Verification items for the finished model (mm, model axes). A direction names the side the tool comes from. Round coordinates to 2 decimals unless told otherwise and drop trailing zeros. Loops run counter-clockwise (first coordinate to the right, second up) from the corner with the lowest first, then second, coordinate; pieces in that order, holes last. Notation, with made-up numbers: (-10.5, 32.25) - (16.5, 32.25) arc R9 cw to (16.5, 40.25) - close; hole circle Ø5 at (75, 64.5). An arc over 180 degrees is marked (long way). Use CSV: the item, a comma, the result in double quotes.
```python
from build123d import *

# Parameters (mm, degrees)
F0_W     = 80
F0_H     = 19
F0_R     = 2.55
F1_DEPTH = 19
F2_R     = 5
F3_DEPTH = 4.5


with BuildPart() as f1:
    # F0 (on Top) → F1 (new body)
    with BuildSketch(Plane.XY):
        Rectangle(F0_W, F0_H)
        with Locations((-30, 0)):
            Circle(F0_R, mode=Mode.SUBTRACT)
        with Locations((-10, 0)):
            Circle(F0_R, mode=Mode.SUBTRACT)
        with Locations((10, 0)):
            Circle(F0_R, mode=Mode.SUBTRACT)
        with Locations((30, 0)):
            Circle(F0_R, mode=Mode.SUBTRACT)
    extrude(amount=F1_DEPTH)

    # F2 (on face) → F3 (cut)
    with BuildSketch(Plane.XY.offset(19)):
        with Locations((-30, 0)):
            Circle(F2_R)
        with Locations((-10, 0)):
            Circle(F2_R)
        with Locations((10, 0)):
            Circle(F2_R)
        with Locations((30, 0)):
            Circle(F2_R)
    extrude(amount=-F3_DEPTH, mode=Mode.SUBTRACT)


solid = f1.part
```
1) Mould release check, pull along X, two halves, no side actions. Record for faces 3 (the face through (-40, 0, 9)), 4 (the face through (-28, -2, 14.5)), 5 (the face through (40, 0, 9)): +X half, -X half, draft (parallel to the pull), parting line (faces both ways), or undercut.
Returned:
face 3,"-X half"
face 4,"undercut"
face 5,"+X half"
2) Cross-section at B-B, the plane z = 7. Record the cut outline in (x, y), then the cut area to 3 significant figures.
Returned:
outline,"(-40, -9.5) - (40, -9.5) - (40, 9.5) - (-40, 9.5) - close; hole circle Ø5.1 at (-30, 0); hole circle Ø5.1 at (-10, 0); hole circle Ø5.1 at (10, 0); hole circle Ø5.1 at (30, 0)"
area,"1,440 mm²"
3) Cross-section at D-D, the plane y = 0. Count the separate pieces of the cut face and the enclosed holes in it, then the cut area to 3 significant figures.
Returned:
separate pieces,"5"
enclosed holes,"0"
area,"1,040 mm²"
4) Cross-section at A-A, the plane x = 30. Record the cut outline in (y, z).
Returned:
outline,"(-9.5, 0) - (-2.55, 0) - (-2.55, 14.5) - (-5, 14.5) - (-5, 19) - (-9.5, 19) - close; (2.55, 0) - (9.5, 0) - (9.5, 19) - (5, 19) - (5, 14.5) - (2.55, 14.5) - close"
5) Access from +Z, -Z, +X, -X, +Y, -Y to the whole of each face (thin tool, end or side, straight path). Record for faces 1 (the face through (12, -2, 14.5)), 2 (the face through (27.452, 0.112, 7.148)).
Returned:
face 1,"+Z"
face 2,"+Z, -Z"
6) Cross-section at C-C, the plane x = -26. Record the cut outline in (y, z), then the cut area to 3 significant figures.
Returned:
outline,"(-9.5, 0) - (9.5, 0) - (9.5, 19) - (3, 19) - (3, 14.5) - (-3, 14.5) - (-3, 19) - (-9.5, 19) - close"
area,"334 mm²"
7) Thickness scan on probe 1 along X at (y, z) = (0, 11); probe 2 along Y at (x, z) = (10, 7.75); probe 3 along Y at (x, z) = (30, 16.5). Record the ranges inside material, lowest first. Write a range as [from, to].
Returned:
probe 1,"x = [-40, -32.55], [-27.45, -12.55], [-7.45, 7.45], [12.55, 27.45], [32.55, 40]"
probe 2,"y = [-9.5, -2.55], [2.55, 9.5]"
probe 3,"y = [-9.5, -5], [5, 9.5]"
8) Gauge pin test, flat ends, axial feed: pin 1 Ø4 at (x, y) = (10, 0) entering from -Z; pin 2 Ø6 at (x, y) = (-10, 0) entering from +Z. Record the tip position at first contact, or that the pin passes through.
Returned:
pin 1,"passes through"
pin 2,"stops at z = 14.5"
